Autodesk Inventor part; units mm, degrees
ref_plane "YZ Plane" through (0, 0, 0) normal (1, 0, 0) x (0, 1, 0)
ref_plane "XZ Plane" through (0, 0, 0) normal (0, 1, 0) x (-1, 0, 0)
ref_plane "XY Plane" through (0, 0, 0) normal (0, 0, 1) x (1, 0, 0)
sketch "Skizze1" plane through (0, 0, 0) normal (0, 1, 0) x (-1, 0, 0)
  line L0 (174.5, 174.5) -> (-174.5, 174.5)
  line L1 (-174.5, 174.5) -> (-174.5, -174.5)
  line L2 (-174.5, -174.5) -> (174.5, -174.5)
  line L3 (174.5, -174.5) -> (174.5, 174.5)
  line L4 (174.5, 174.5) -> (-174.5, -174.5) construction
  line L5 (-174.5, 174.5) -> (174.5, -174.5) construction
  line L6 (244.3, 0) -> (-244.3, 0) construction
  line L7 (0, -244.3) -> (0, 244.3) construction
  arc A0 (10, -167) -> (-10, -167) centre (0, -167) ccw
  arc A1 (85, -167) -> (65, -167) centre (75, -167) ccw
  arc A2 (-65, -167) -> (-85, -167) centre (-75, -167) ccw
  line L8 (85, -167) -> (85, -174.5)
  line L9 (65, -167) -> (65, -174.5)
  line L10 (10, -167) -> (10, -174.5)
  line L11 (-10, -167) -> (-10, -174.5)
  line L12 (-65, -167) -> (-65, -174.5)
  line L13 (-85, -167) -> (-85, -174.5)
  line L14 (-65, -174.5) -> (-85, -174.5)
  line L15 (10, -174.5) -> (-10, -174.5)
  line L16 (85, -174.5) -> (65, -174.5)
  line L17 (40, 174.5) -> (-40, 174.5)
  line L18 (-40, 174.5) -> (-40, 157.5)
  line L19 (-40, 157.5) -> (40, 157.5)
  line L20 (40, 157.5) -> (40, 174.5)
  arc A3 (65, 167) -> (85, 167) centre (75, 167) ccw
  arc A4 (-85, 167) -> (-65, 167) centre (-75, 167) ccw
  line L21 (85, 167) -> (85, 174.5)
  line L22 (65, 167) -> (65, 174.5)
  line L23 (-65, 167) -> (-65, 174.5)
  line L24 (-85, 167) -> (-85, 174.5)
  line L25 (-65, 174.5) -> (-85, 174.5)
  line L26 (85, 174.5) -> (65, 174.5)
  point P0 (0, 0)
  dimension "d0" = 349
  dimension "d1" = 349
  dimension "d2" = 20
  dimension "d3" = 17.5
  dimension "d4" = 150
  dimension "d5" = 17
  dimension "d6" = 80
extrude "Extrusion1" add sketch "Skizze1" along normal blind 2 contours L3 L2 L8 A1 L9 L10 A0 L11 L12 A2 L13 L1 L0 L24 A4 L23 L18 L19 L20 L22 A3 L21
fillet "Rundung1" radius 1.5 28 edges at (-129.75, 2, 174.5) (-75, 2, 157) (-65, 2, 170.75) (-85, 2, 170.75) (-52.5, 2, 174.5) (-40, 2, 166) (0, 2, 157.5) (40, 2, 166) (52.5, 2, 174.5) (75, 2, 157) (85, 2, 170.75) (65, 2, 170.75) (129.75, 2, 174.5) (174.5, 2, 0) (129.75, 2, -174.5) (65, 2, -170.75) (85, 2, -170.75) (75, 2, -157) (37.5, 2, -174.5) (-10, 2, -170.75) (10, 2, -170.75) (0, 2, -157) (-37.5, 2, -174.5) (-85, 2, -170.75) (-65, 2, -170.75) (-75, 2, -157) (-129.75, 2, -174.5) (-174.5, 2, 0)
properties part number "Silicon-Heater (350mm)" material "Gummi, Silikon"
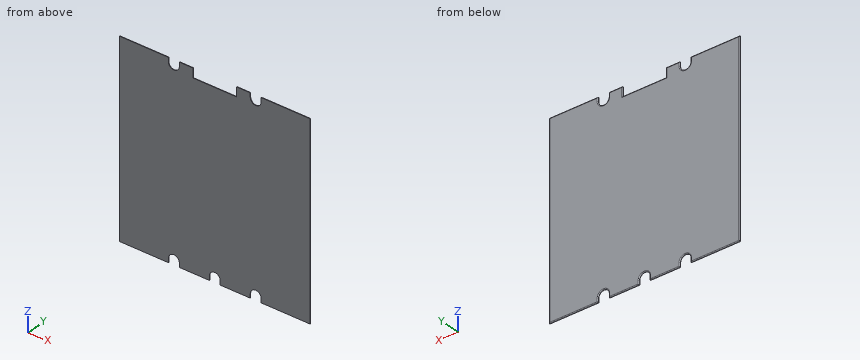
Work out the finished part from the listing and answer in its coordinate system (mm). Round coordinates to 2 decimals unless told otherwise and drop trailing zeros. Write each loop counter-clockwise with the first axis right and the second up, starting at its lowest first coordinate (ties: lowest second). Pieces come first, ordered by that corner, then holes. Notation, with made-up numbers: (-1.5, 81) -> (42.5, 81) arc R22 ccw to (42.5, 102) -> close; hole circle Ø3 at (79.25, 53.25). An arc over 180 degrees is marked (long way). Answer as CSV lines item,"result". Start each with the question number.
(1) The part is cut by section B-B, the plane y = 1.65. Give the vertices of the cut face in (x, z).
(2) The part is cut by section C-C, the plane x = 75. Give the vertices of the cut face in (y, z), then the cut area to 3 significant figures.
(3) The part is cut by section A-A, the plane x = 0. Give the vertices of the cut face in (y, z).
(4) Each of these flat-tipped pins is pushed along its axis until it touches: pin 1 (1 mm diameter, centred on x = -121, y = 1, fed in from -Z); pin 2 (0.6 mm diameter, centred on x = 16, y = 0.5, fed in from +Z). Where does it stop, or does it pass through?
(5) Find the intervals of material crossed by probe 1 along Z at (x, y) = (-93, 1); probe 2 along Z at (x, y) = (32, 1.3), in increasing order.
Output values:
1,outline,"(-173.96, -173.96) -> (-85.54, -173.96) -> (-85.54, -167) arc R10.54 cw to (-64.46, -167) -> (-64.46, -173.96) -> (-10.54, -173.96) -> (-10.54, -167) arc R10.54 cw to (10.54, -167) -> (10.54, -173.96) -> (64.46, -173.96) -> (64.46, -167) arc R10.54 cw to (85.54, -167) -> (85.54, -173.96) -> (173.96, -173.96) -> (173.96, 173.96) -> (85.54, 173.96) -> (85.54, 167) arc R10.54 cw to (64.46, 167) -> (64.46, 173.96) -> (40.54, 173.96) -> (40.54, 156.96) -> (-40.54, 156.96) -> (-40.54, 173.96) -> (-64.46, 173.96) -> (-64.46, 167) arc R10.54 cw to (-85.54, 167) -> (-85.54, 173.96) -> (-173.96, 173.96) -> close"
2,outline,"(0, -157) -> (0.5, -157) arc R1.5 ccw to (2, -155.5) -> (2, 155.5) arc R1.5 ccw to (0.5, 157) -> (0, 157) -> close"
2,area,"627 mm²"
3,outline,"(0, -157) -> (0.5, -157) arc R1.5 ccw to (2, -155.5) -> (2, 156) arc R1.5 ccw to (0.5, 157.5) -> (0, 157.5) -> close"
4,pin 1,"stops at z = -174.5"
4,pin 2,"stops at z = 157.5"
5,probe 1,"z = -174.41 to 174.41"
5,probe 2,"z = -174.27 to 157.27"
